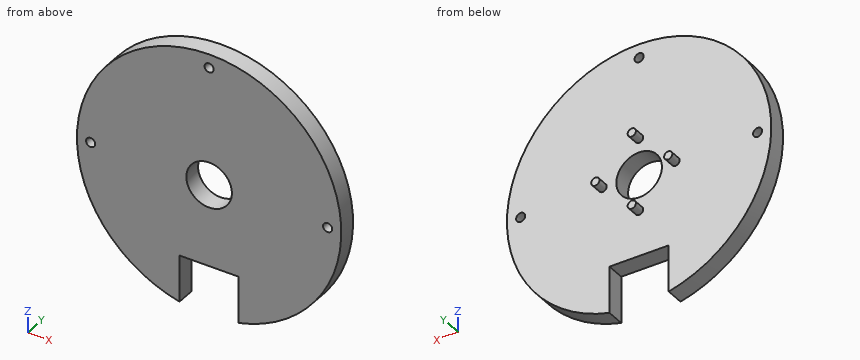
```python
from build123d import *

# Parameters (mm, degrees)
SKETCH1_R           = 29
BOSS_EXTRUDE1_DEPTH = 5
SKETCH3_W           = 13
SKETCH3_H           = 11
CUT_EXTRUDE1_DEPTH  = 10
SKETCH4_R           = 0.9
BOSS_EXTRUDE2_DEPTH = 2.5
SKETCH7_R           = 5
CUT_EXTRUDE4_DEPTH  = 5
SKETCH11_R          = 1
CUT_EXTRUDE6_DEPTH  = 5
SKETCH12_R          = 29
CUT_EXTRUDE7_DEPTH  = 1


with BuildPart() as part:
    # Sketch1 → Boss-Extrude1 (new body)
    with BuildSketch(Plane(origin=(0, 0, 0), x_dir=(1, 0, 0), z_dir=(0, 1, 0))):
        with Locations(Location((0, 0, 0), (0, 0, 270))):
            Circle(SKETCH1_R)
    extrude(amount=BOSS_EXTRUDE1_DEPTH)

    # Sketch3 → Cut-Extrude1 (cut)
    with BuildSketch(Plane(origin=(0, 5, 0), x_dir=(1, 0, 0), z_dir=(0, 1, 0))):
        with Locations((0, 23.5)):
            Rectangle(SKETCH3_W, SKETCH3_H)
    extrude(amount=-CUT_EXTRUDE1_DEPTH, mode=Mode.SUBTRACT)

    # Sketch4 → Boss-Extrude2 (add)
    with BuildSketch(Plane(origin=(0, 5, 0), x_dir=(1, 0, 0), z_dir=(0, 1, 0))):
        with Locations(Location((8, 0, 0), (0, 0, 270))):
            Circle(SKETCH4_R)
        with Locations(Location((-8, 0, 0), (0, 0, 270))):
            Circle(SKETCH4_R)
        with Locations(Location((0, 8, 0), (0, 0, 270))):
            Circle(SKETCH4_R)
        with Locations(Location((0, -8, 0), (0, 0, 270))):
            Circle(SKETCH4_R)
    extrude(amount=BOSS_EXTRUDE2_DEPTH)

    # Sketch7 → Cut-Extrude4 (cut)
    with BuildSketch(Plane(origin=(0, 5, 0), x_dir=(1, 0, 0), z_dir=(0, 1, 0))):
        with Locations(Location((0, 0, 0), (0, 0, 270))):
            Circle(SKETCH7_R)
    extrude(amount=-CUT_EXTRUDE4_DEPTH, mode=Mode.SUBTRACT)

    # Sketch11 → Cut-Extrude6 (cut)
    with BuildSketch(Plane(origin=(0, 5, 0), x_dir=(1, 0, 0), z_dir=(0, 1, 0))):
        with Locations(Location((-26, 0, 0), (0, 0, 270))):
            Circle(SKETCH11_R)
        with Locations(Location((0, -26, 0), (0, 0, 270))):
            Circle(SKETCH11_R)
        with Locations(Location((26, 0, 0), (0, 0, 270))):
            Circle(SKETCH11_R)
    extrude(amount=-CUT_EXTRUDE6_DEPTH, mode=Mode.SUBTRACT)

    # Sketch12 → Cut-Extrude7 (cut)
    with BuildSketch(Plane(origin=(0, 0, 0), x_dir=(-1, 0, 0), z_dir=(0, -1, 0))):
        Circle(SKETCH12_R)
    extrude(amount=-CUT_EXTRUDE7_DEPTH, mode=Mode.SUBTRACT)


solid = part.part
```
Verification items for the finished model (mm, model axes). Round coordinates to 2 decimals unless told otherwise and drop trailing zeros. Loops run counter-clockwise (first coordinate to the right, second up) from the corner with the lowest first, then second, coordinate; pieces in that order, holes last. Notation, with made-up numbers: (0.5, 25.5) -> (24.5, 25.5) arc R30 cw to (24.5, 59.5) -> close; hole circle Ø8 at (-13, 17.25). An arc over 180 degrees is marked (long way). Answer as a JSON object with one key per item and string values.
Q1. Scan lines: line 1 (X direction, y = 2.5, z = 0); line 2 (Y direction, x = 8, z = -4.5); line 3 (X direction, y = 4.25, z = -4). Record each from-to range of solid material in increasing order. Write a range as from..to.
Data:
{"line 1": "x = -29..-27, -25..-5, 5..25, 27..29", "line 2": "y = 1..5", "line 3": "x = -28.72..-3, 3..28.72"}
Q2. Section check A-A (y = 2.5). Record the boundary of the cut face in (x, z), then the cut area to 3 significant figures.
Data:
{"outline": "(-6.5, -28.26) -> (-6.5, -18) -> (6.5, -18) -> (6.5, -28.26) arc R29 ccw (long way) to start; hole circle Ø2 at (-26, 0); hole circle Ø10 at (0, 0); hole circle Ø2 at (0, 26); hole circle Ø2 at (26, 0)", "area": "2,410 mm2"}
Q3. Go/stop test with flat-tipped pins: P1, Ø1, axis at x = 16.5, y = 5, coming from the -Z side; P2, Ø1.2, axis at y = 3, z = -25.5, coming from the +X side; P3, Ø1.2, axis at y = 3, z = -23.5, coming from the -X side; P4, Ø17, axis at x = 7.5, z = 11, coming from the +Y side. Record where each tip stops, or that it passes through.
Data:
{"P1": "stops at z = -24.19", "P2": "stops at x = 14.87", "P3": "stops at x = -17.79", "P4": "stops at y = 7.5"}
Q4. Section check D-D (x = 26). Record the boundary of the cut face in (y, z).
Data:
{"outline": "(1, -12.85) -> (5, -12.85) -> (5, -1) -> (1, -1) -> close; (1, 1) -> (5, 1) -> (5, 12.85) -> (1, 12.85) -> close"}
Q5. Section check C-C (z = 4). Record the boundary of the cut face in (x, y), then the cut area to 3 significant figures.
Data:
{"outline": "(-28.72, 1) -> (-3, 1) -> (-3, 5) -> (-28.72, 5) -> close; (3, 1) -> (28.72, 1) -> (28.72, 5) -> (3, 5) -> close", "area": "206 mm2"}
Q6. Section check B-B (x = 0). Record the boundary of the cut face in (y, z).
Data:
{"outline": "(1, -18) -> (5, -18) -> (5, -8.9) -> (7.5, -8.9) -> (7.5, -7.1) -> (5, -7.1) -> (5, -5) -> (1, -5) -> close; (1, 5) -> (5, 5) -> (5, 7.1) -> (7.5, 7.1) -> (7.5, 8.9) -> (5, 8.9) -> (5, 25) -> (1, 25) -> close; (1, 27) -> (5, 27) -> (5, 29) -> (1, 29) -> close"}
